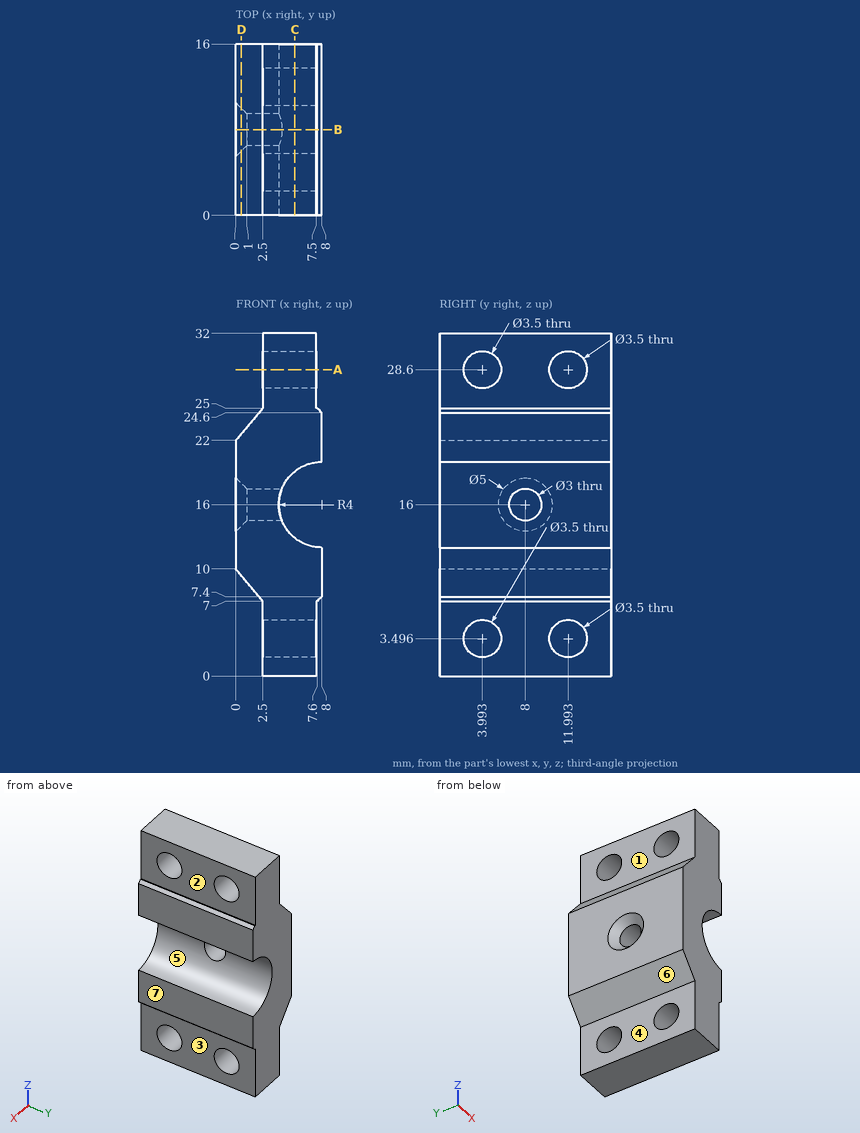
Could you check a few things on this drawing? It's one solid part, dimensions in mm from its lowest x, y, z. A direction names the side the tool comes from. Round coordinates to 2 decimals unless told otherwise and drop trailing zeros. Write each loop counter-clockwise with the first axis right and the second up, starting at its lowest first coordinate (ties: lowest second). Pieces come first, ordered by that corner, then holes. Notation, with made-up numbers: (66, -35.5) -> (70, -35.5) arc R18 cw to (70, -29.5) -> close; hole circle Ø10 at (82, 2). An arc over 180 degrees is marked (long way). Use one line per item in the form item = value. Start each with the question number.
Q1. Imagine slicing it at B-B (y = 8). Please give me the cut outline in (x, z).
Q2. Imagine slicing it at C-C (x = 5.5). Please give me the cut outline in (y, z).
Q3. Imagine slicing it at D-D (x = 0.5). Please give me the cut outline in (y, z).
Q4. Which directions (+Z, -Z, +X, -X, +Y, -Y) give clear straight access to the entire face, cutting with the end or side of a thin tool? Please do the marked faces 1, 2, 3 and 4.
Q5. I'm going to push flat-ended pins straight in: P1, Ø4, axis at y = 11, z = 27.5, coming from the -X side; P2, Ø4, axis at y = 11.99, z = 3.5, coming from the +X side; P3, Ø5, axis at y = 8, z = 16, coming from the +X side. Where does each tip first touch, or does it pass through?
Q6. If I drill on probe 1 along Y at (x, z) = (5.05, 28.6); probe 2 along Y at (x, z) = (6, 29.5) (1 decimal); probe 3 along Y at (x, z) = (3.1, 16), over which ranges is the centre line in solid material (lowest first)? Write a range as [from, to].
Q7. We'd pull the mould along Z, two halves only. Please class the marked faces 5, 6 and 7: +Z half, -Z half, draft (parallel to the pull), parting line (faces both ways), or undercut.
Q8. Imagine slicing it at A-A (z = 28.6). Please give me the cut outline in (x, y).
Worked out:
q1.outline = (0, 10) -> (2.5, 7) -> (2.5, 0) -> (7.5, 0) -> (7.5, 7) -> (7.6, 7) -> (8, 7.4) -> (8, 12) arc R4 cw to (4.29, 14.5) -> (1, 14.5) -> (0, 13.5) -> close; (0, 18.5) -> (1, 17.5) -> (4.29, 17.5) arc R4 cw to (8, 20) -> (8, 24.6) -> (7.6, 25) -> (7.5, 25) -> (7.5, 32) -> (2.5, 32) -> (2.5, 25) -> (0, 22) -> close
q2.outline = (0, 0) -> (16, 0) -> (16, 12.88) -> (0, 12.88) -> close; (0, 19.12) -> (16, 19.12) -> (16, 32) -> (0, 32) -> close; hole circle Ø3.5 at (3.99, 3.5); hole circle Ø3.5 at (3.99, 28.6); hole circle Ø3.5 at (11.99, 3.5); hole circle Ø3.5 at (11.99, 28.6)
q3.outline = (0, 9.4) -> (16, 9.4) -> (16, 22.6) -> (0, 22.6) -> close; hole circle Ø4 at (8, 16)
q4.face_1 = +Z, -X, +Y, -Y
q4.face_2 = +Z, +X, +Y, -Y
q4.face_3 = -Z, +X, +Y, -Y
q4.face_4 = -Z, -X, +Y, -Y
q5.P1 = 2.5
q5.P2 = 7.5
q5.P3 = 4.88
q6.probe_1 = [0, 2.24], [5.74, 10.24], [13.74, 16]
q6.probe_2 = [0, 2.5], [5.5, 10.5], [13.5, 16]
q6.probe_3 = [0, 6.5], [9.5, 16]
q7.face_5 = undercut
q7.face_6 = -Z half
q7.face_7 = draft
q8.outline = (2.5, 0) -> (7.5, 0) -> (7.5, 2.24) -> (2.5, 2.24) -> close; (2.5, 5.74) -> (7.5, 5.74) -> (7.5, 10.24) -> (2.5, 10.24) -> close; (2.5, 13.74) -> (7.5, 13.74) -> (7.5, 16) -> (2.5, 16) -> close
